Part model, mm, in its own coordinate system. Coordinates: 2 decimals unless noted, no trailing zeros. Loops run counter-clockwise (first coordinate to the right, second up) from the corner with the lowest first, then second, coordinate; pieces in that order, holes last. Notation, with made-up numbers: (-38.5, -6.75) -> (16.5, -6.75) arc R36 cw to (16.5, 31.25) -> close; hole circle Ø8 at (15, -17). An arc over 180 degrees is marked (long way). Use one line per item in the form item = value. Start each with the question number.
(1) Band-saw the part on B-B on y = 57.15. Give the cut face in (x, z), then the cut area to 3 significant figures.
(2) Pin check, flat tips, straight feed: P1, Ø3, axis at y = 96.5, z = 5.5, coming from the -X side; P2, Ø8.5, axis at x = 19.05, y = 57.15, coming from the -Z side; P3, Ø2, axis at x = 14.5, z = 4, coming from the +Y side; P4, Ø1, axis at x = 16, z = 1.5, coming from the +Y side. Stop position of each tip, or through.
(3) Band-saw the part on D-D on x = 34. Give the cut face in (y, z), then the cut area to 3 significant figures.
(4) Band-saw the part on A-A on x = 19.05. Give the cut face in (y, z).
(5) Drill centre lines: L1, parallel to Y at x = 19.05, z = 2; L2, parallel to X at y = 107.5, z = 3.25; L3, parallel to Y at x = 35.5, z = 3.25. Where is each one in solid material? Low to high. Write a range as [from, to].
(6) Band-saw the part on C-C on z = 2.5. Count the separate pieces of the cut face and the enclosed holes in it, then the cut area to 3 significant figures.
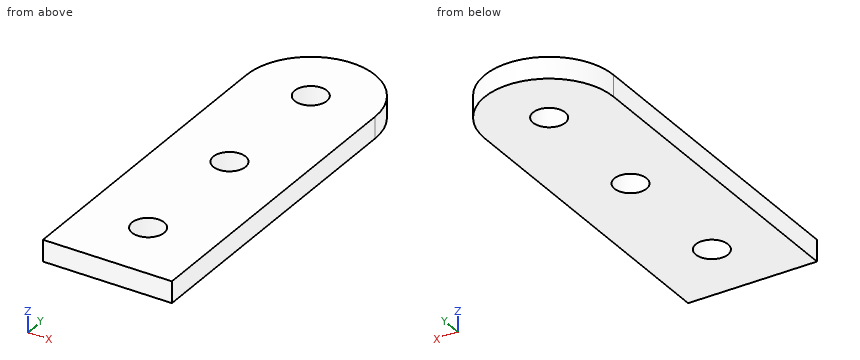
```python
from build123d import *

# Parameters (mm, degrees)
F0_W     = 38.1
F0_H     = 95.25
F1_DEPTH = 6.35
F3_D     = 9.525


with BuildPart() as f1:
    # F0 (on Top) → F1 (new body)
    with BuildSketch(Plane.XY):
        with Locations((19.05, 47.625)):
            Rectangle(F0_W, F0_H)
        with BuildLine():
            ThreePointArc((38.1, 95.25), (19.05, 114.3), (0, 95.25))
            Line((0, 95.25), (38.1, 95.25))
        make_face()
    extrude(amount=F1_DEPTH)

    # F3 (through all)
    with Locations(Plane.XY.offset(6.35)):
        with Locations((19.05, 95.25), (19.05, 57.15), (19.05, 19.05)):
            Hole(F3_D / 2)


solid = f1.part
```
A:
q1.outline = (0, 0) -> (14.29, 0) -> (14.29, 6.35) -> (0, 6.35) -> close; (23.81, 0) -> (38.1, 0) -> (38.1, 6.35) -> (23.81, 6.35) -> close
q1.area = 181 mm²
q2.P1 = 0
q2.P2 = through
q2.P3 = 113.97
q2.P4 = 114.13
q3.outline = (0, 0) -> (107.06, 0) -> (107.06, 6.35) -> (0, 6.35) -> close
q3.area = 680 mm²
q4.outline = (0, 0) -> (14.29, 0) -> (14.29, 6.35) -> (0, 6.35) -> close; (23.81, 0) -> (52.39, 0) -> (52.39, 6.35) -> (23.81, 6.35) -> close; (61.91, 0) -> (90.49, 0) -> (90.49, 6.35) -> (61.91, 6.35) -> close; (100.01, 0) -> (114.3, 0) -> (114.3, 6.35) -> (100.01, 6.35) -> close
q5.L1 = [0, 14.29], [23.81, 52.39], [61.91, 90.49], [100.01, 114.3]
q5.L2 = [4.46, 33.64]
q5.L3 = [0, 104.86]
q6.separate_pieces = 1
q6.enclosed_holes = 3
q6.area = 3,990 mm²
